Part print with two shaded views. Sizes in mm from the minimum x, y, z corner. Round coordinates to 2 decimals unless told otherwise and drop trailing zeros. Write each loop counter-clockwise with the first axis right and the second up, starting at its lowest first coordinate (ties: lowest second). Pieces come first, ordered by that corner, then holes. Notation, with made-up numbers: M 38.25,-35 L 68.25,-35 A22 ccw 68.25,3 Z; hole C 56.5,38 d6. An arc over 180 degrees is marked long. One line per question, with ' | ' between items. Start each with the question number.
1) Drop a flat-ended pin along its axis: pin 1 Ø4.5 at (y, z) = (4, 5) entering from -X. Give the stop position or say it passes through.
2) Wall check: probe 1 along Y at (x, z) = (2.7, 5); probe 2 along X at (y, z) = (3.5, 77). Give the ranges that are in metal, low to high. Write a range as [from, to].
3) Saw through at B-B (z = 5). List the corners of the cut face in (x, y), plus the area to 3 significant figures.
4) Saw through at A-A (y = 4). List the corners of the cut face in (x, z), plus the area to 3 significant figures.
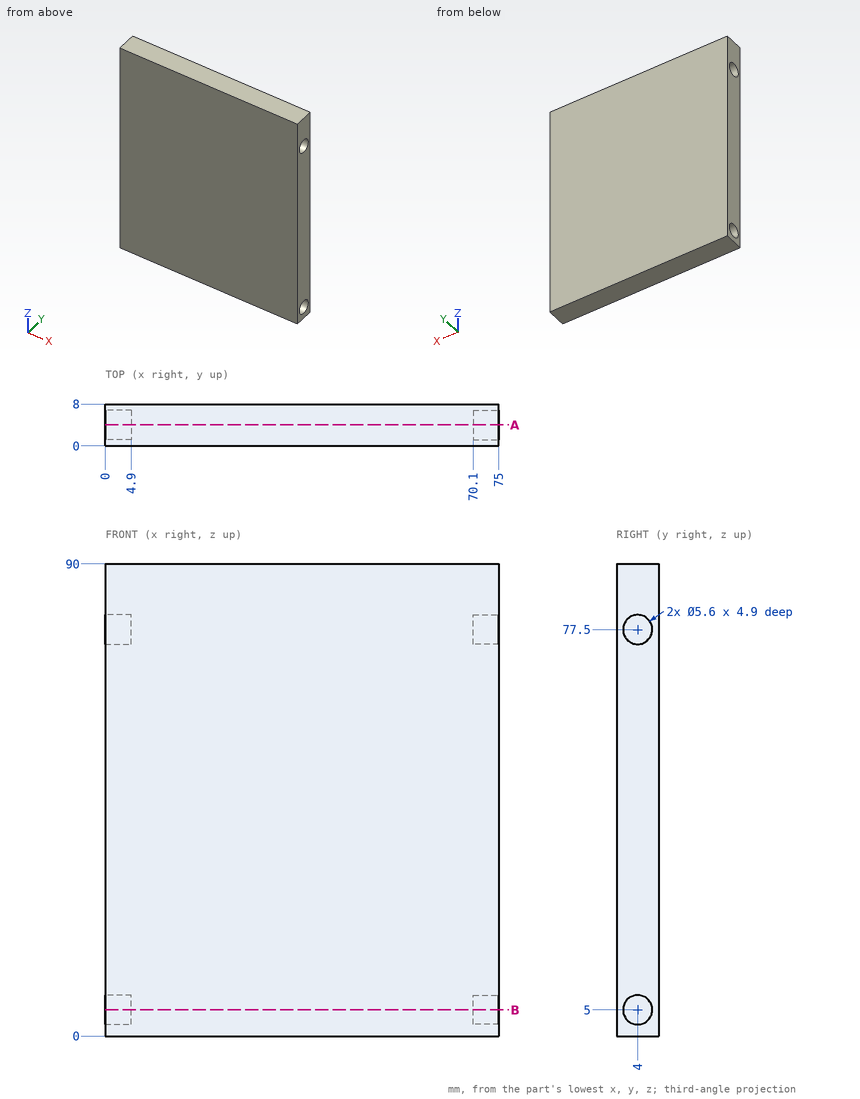
Answer key:
1) pin 1: stops at x = 4.9
2) probe 1: y = [0, 1.2], [6.8, 8] | probe 2: x = [4.9, 70.1]
3) outline: M 0,0 L 75,0 L 75,1.2 L 70.1,1.2 L 70.1,6.8 L 75,6.8 L 75,8 L 0,8 L 0,6.8 L 4.9,6.8 L 4.9,1.2 L 0,1.2 Z | area: 545 mm2
4) outline: M 0,0 L 75,0 L 75,2.2 L 70.1,2.2 L 70.1,7.8 L 75,7.8 L 75,74.7 L 70.1,74.7 L 70.1,80.3 L 75,80.3 L 75,90 L 0,90 L 0,80.3 L 4.9,80.3 L 4.9,74.7 L 0,74.7 L 0,7.8 L 4.9,7.8 L 4.9,2.2 L 0,2.2 Z | area: 6,640 mm2
